```python
from build123d import *

# Parameters (mm, degrees)
SKETCH1_R           = 2.9
SKETCH1_R_2         = 4.064
BOSS_EXTRUDE1_DEPTH = 2.54
SKETCH2_R           = 2.9
BOSS_EXTRUDE2_DEPTH = 2.54


with BuildPart() as part:
    # Sketch1 → Boss-Extrude1 (new body)
    with BuildSketch(Plane.XY):
        with BuildLine():
            Line((0, 12.7), (17.018, 12.7))
            ThreePointArc((17.018, 12.7), (23.368, 6.35), (17.018, 0))
            Line((17.018, 0), (0, 0))
            ThreePointArc((0, 0), (-6.35, 6.35), (0, 12.7))
        make_face()
        with Locations((-2.54, 6.35)):
            Circle(SKETCH1_R, mode=Mode.SUBTRACT)
        with Locations((17.272, 6.35)):
            Circle(SKETCH1_R_2, mode=Mode.SUBTRACT)
    extrude(amount=BOSS_EXTRUDE1_DEPTH)

    # Sketch2 → Boss-Extrude2 (add)
    with BuildSketch(Plane.XY.offset(2.54)):
        with BuildLine():
            ThreePointArc((0, 0), (4.490128061, 1.859871939), (6.35, 6.35))
            ThreePointArc((6.35, 6.35), (4.490128061, 10.840128061), (0, 12.7))
            ThreePointArc((0, 12.7), (-6.35, 6.35), (0, 0))
        make_face()
        with Locations((-2.54, 6.35)):
            Circle(SKETCH2_R, mode=Mode.SUBTRACT)
    extrude(amount=BOSS_EXTRUDE2_DEPTH)


solid = part.part
```
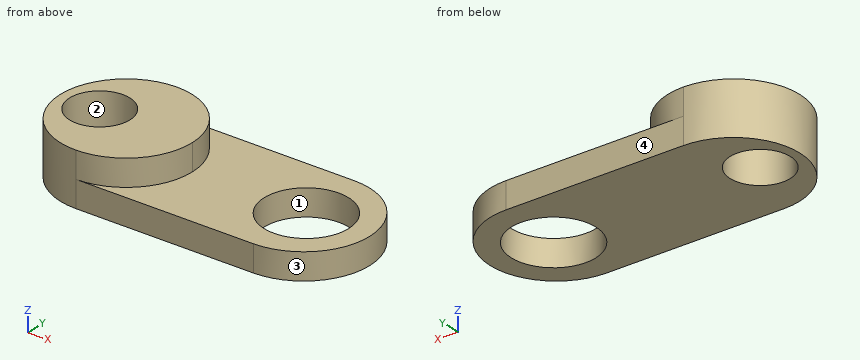
Could you check a few things on this model? Use its own coordinates, in mm. Face numbers are marked on the shaded views. Coordinates: 2 decimals unless noted, no trailing zeros. Loops run counter-clockwise (first coordinate to the right, second up) from the corner with the lowest first, then second, coordinate; pieces in that order, holes last. Notation, with made-up numbers: M 2.25,-22 L 17.25,-22 A25 cw 17.25,-9 Z; hole C 18.5,39.25 d10. An arc over 180 degrees is marked long. Put each result on its own line as item: value. Start each with the question number.
(1) Will these pins go through, and if not, where does the flat tip stop? P1, Ø1, axis at y = 10.5, z = 2.5, coming from the +X side; P2, Ø1, axis at x = 20, z = 1, coming from the +Y side; P3, Ø1, axis at x = 16, z = 3, coming from the -Y side.
(2) Suppose I cut it at A-A on x = -2.54. Please give me the cut outline in (y, z), then the cut area to 3 significant figures.
(3) Suppose I cut it at C-C on z = 3.15. Please give me the cut outline in (x, y), then the cut area to 3 significant figures.
(4) I need wall thicknesses on line 1 (X direction, y = 5.5, z = 0.65); line 2 (Z direction, x = 16.75, y = 0.5); line 3 (Y direction, x = -1.5, z = 0.85). Which ranges of each line are inside material? Lowest first, please. Write a range as from..to.
(5) Suppose I cut it at D-D on x = 2. Please give me the cut outline in (y, z).
(6) Suppose I cut it at B-B on z = 0.75. Please give me the cut outline in (x, y), then the cut area to 3 significant figures.
(7) Thinking about a two-plate mould opening in X: for the marked faces 1, 2, 3 and 4, which applies, pulls with the +X half, pulls with the -X half, needs draft (parallel to the pull), parting line crosses it, or undercut?
Solutions:
1. P1: stops at x = 22.21
1. P2: stops at y = 12.19
1. P3: stops at y = 0
2. outline: M 0.53,0 L 3.45,0 L 3.45,5.08 L 0.53,5.08 Z; M 9.25,0 L 12.17,0 L 12.17,5.08 L 9.25,5.08 Z
2. area: 29.7 mm2
3. outline: C 0,6.35 d12.7; hole C -2.54,6.35 d5.8
3. area: 100 mm2
4. line 1: x = -6.29..-5.31, 0.23..13.3, 21.25..23.31
4. line 2: z = 0..2.54
4. line 3: y = 0.18..3.64, 9.06..12.52
5. outline: M 0,0 L 12.7,0 L 12.7,2.54 L 12.38,2.54 L 12.38,5.08 L 0.32,5.08 L 0.32,2.54 L 0,2.54 Z
6. outline: M 0,0 L 17.02,0 A6.35 ccw 17.02,12.7 L 0,12.7 A6.35 ccw Z; hole C -2.54,6.35 d5.8; hole C 17.27,6.35 d8.13
6. area: 264 mm2
7. face 1: undercut
7. face 2: undercut
7. face 3: pulls with the +X half
7. face 4: needs draft
